Autodesk Inventor part; units mm, degrees
ref_plane "YZ Plane" through (0, 0, 0) normal (1, 0, 0) x (0, 1, 0)
ref_plane "XZ Plane" through (0, 0, 0) normal (0, 1, 0) x (-1, 0, 0)
ref_plane "XY Plane" through (0, 0, 0) normal (0, 0, 1) x (1, 0, 0)
sketch "Sketch1" plane through (0, 0, 0) normal (0, 0, 1) x (1, 0, 0)
  line L0 (-125, -70) -> (125, -70)
  line L1 (125, -70) -> (125, 70)
  line L2 (125, 70) -> (-125, 70)
  line L3 (-125, 70) -> (-125, -70)
  line L4 (-125, -70) -> (125, 70) construction
  line L5 (125, -70) -> (-125, 70) construction
  point P0 (0, 0)
  dimension "d0" = 250
  dimension "d1" = 140
extrude "Extrusion1" add sketch "Sketch1" along normal blind 38
sketch "Sketch2" plane through (0, 0, 38) normal (0, 0, 1) x (1, 0, 0)
  line L0 (125, -70) -> (125, 70)
  line L1 (125, 70) -> (-125, 70)
  line L2 (-125, 70) -> (-125, -70)
  line L3 (-125, -70) -> (125, -70)
  line L4 (-125, -70) -> (125, -70)
  arc A0 (85, -70) -> (-85, -70) centre (0, -175.4167) ccw
  line L5 (53.4733, -40) -> (-37.6413, -40) construction
  point P0 (0, 0)
  point P1 (85, -70)
  dimension "d5" = 40
  dimension "d114" = 30
extrude "Extrusion2" cut sketch "Sketch2" against normal through all contours L3 A0
fillet "Fillet1" radius 40 2 edges at (125, 70, 19) (-125, 70, 19)
sketch "Sketch3" plane through (0, 0, 38) normal (0, 0, 1) x (1, 0, 0)
  point P0 (0, 0)
  point P1 (-68.7955, 12.1981)
hole "Hole1" at (-68.7955, 12.1981, 38) direction (0, 0, -1) diameter 10 end through all countersink diameter 16 countersink angle 90
sketch "Sketch4" plane through (0, 0, 38) normal (0, 0, 1) x (1, 0, 0)
  line L0 (16.3939, 32.185) -> (98.1222, 32.185)
  line L1 (98.1222, 32.185) -> (98.1222, -13.1392)
  line L2 (98.1222, -13.1392) -> (16.3939, -13.1392)
  line L3 (16.3939, -13.1392) -> (16.3939, 32.185)
  point P0 (0, 0)
extrude "Extrusion3" cut sketch "Sketch4" against normal blind 10
properties part number "Demo Covering Queue 2" material "MLBRD"
Geometry: final body of the model. Coordinates: model frame, mm. A direction names the side the tool comes from. Give positions to 0.01 mm unless a question says otherwise; leave off trailing zeros. Order: outer loops, then holes, each group sorted by start corner. A loop starts at its lowest first (then second) coordinate and runs counter-clockwise, first axis right, second up. Notation, with made-up numbers: (28, -25.75) -> (65, -25.75) arc R19 ccw to (65, -17.75) -> close; hole circle Ø6 at (69.25, -21). An arc over 180 degrees is marked (long way). Write each question's results on one line, items separated by ' | '. Start each with the question number.
1) Section B-B (x = 57). Return loops of the section in (y, z) (3 decimals).
2) Set-up query: faces 4 (the flat face through (57, 32.185, 33)), 5 (the flat face through (125, -21, 19)). Return all of +Z, -Z, +X, -X, +Y, -Y with unobstructed straight access to the full face (end or side cutting, diameter ignored); none if empty.
3) Section C-C (z = 9). Return loops of the section in (x, y), then the cut area to 3 significant figures.
4) Draft query along Y for faces 1 (the conical face through (-63.65, 12.87, 35.19)), 2 (the flat face through (-2, 1, 38)), 3 (the cylindrical face through (113.594, 57.972, 19.266)). Return one class per face: pulls with the +Y half, pulls with the -Y half, needs draft (parallel to the pull), parting line crosses it, or undercut.
5) Section A-A (y = -47). Return loops of the section in (x, z), then the cut area to 3 significant figures.
6) Section D-D (x = 94). Return loops of the section in (y, z) (3 decimals), then the cut area to 3 significant figures.
7) First-contact query: pin 1 (4 mm diameter, centred on x = -12, z = 22.5, fed in from -Y); pin 2 (5 mm diameter, centred on x = 44, z = 33, fed in from -Y). Flat tips, straight axial feed; report the tip coordinate or a pass-through.
8) Line query: line 1 (X direction, y = 1, z = 34); line 2 (Y direction, x = -2.5, z = 13); line 3 (X direction, y = -51, z = 20). Output: solid intervals per line, ascending. Write a range as from..to.
Calculated:
1) outline: (-52.581, 0) -> (70, 0) -> (70, 38) -> (32.185, 38) -> (32.185, 28) -> (-13.139, 28) -> (-13.139, 38) -> (-52.581, 38) -> close
2) face 4: +Z | face 5: +Z, -Z, +X, +Y, -Y
3) outline: (-125, -70) -> (-85, -70) arc R135.42 cw to (85, -70) -> (125, -70) -> (125, 30) arc R40 ccw to (85, 70) -> (-85, 70) arc R40 ccw to (-125, 30) -> close; hole circle Ø10 at (-68.8, 12.2) | area: 30,800 mm2
4) face 1: undercut | face 2: needs draft | face 3: pulls with the +Y half
5) outline: (-125, 0) -> (-42.97, 0) -> (-42.97, 38) -> (-125, 38) -> close; (42.97, 0) -> (125, 0) -> (125, 38) -> (42.97, 38) -> close | area: 6,230 mm2
6) outline: (-70, 0) -> (68.974, 0) -> (68.974, 38) -> (32.185, 38) -> (32.185, 28) -> (-13.139, 28) -> (-13.139, 38) -> (-70, 38) -> close | area: 4,830 mm2
7) pin 1: y = -40.73 | pin 2: y = -48.23
8) line 1: -125..16.39, 98.12..125 | line 2: -40.02..70 | line 3: -125..-53.46, 53.46..125
